Part model, mm, in its own coordinate system. A direction names the side the tool comes from. Round coordinates to 2 decimals unless told otherwise and drop trailing zeros. Loops run counter-clockwise (first coordinate to the right, second up) from the corner with the lowest first, then second, coordinate; pieces in that order, holes last. Notation, with made-up numbers: M 49,84 L 90,84 A13 cw 90,106 Z; hole C 67.25,84 d2. An arc over 180 degrees is marked long. Answer as CSV lines item,"result". Start each with the question number.
Item 1: Band-saw the part on B-B (z = -58). Give the cut face in (x, y), and give its area (3 significant figures).
Item 2: Band-saw the part on A-A (y = 0.95). Count the separate pieces of the cut face and the enclosed holes in it, and give its area (3 significant figures).
Item 3: Which spindle directions (+Z, -Z, +X, -X, +Y, -Y) get a long thin tool onto all of the face, cutting with end or side? Do faces 1 (the flat face through (-8.235, 0, -93)), 2 (the flat face through (0, -1.984, -115)), 3 (the flat face through (8.235, 0, -107)). Say none if no direction does.
Item 4: Wall check: line 1 (Z direction, x = -4.5, y = 0.2); line 2 (Z direction, x = 1, y = 0.6); line 3 (X direction, y = 1.45, z = -103). Give the ranges that are in metal, low to high.
Item 5: Drop flat-ended pins along their axis: pin 1 Ø2 at (y, z) = (0.5, -190.5) entering from -X; pin 2 Ø1.5 at (y, z) = (0.5, -86) entering from -X; pin 3 Ø2 at (x, y) = (2.5, 0.5) entering from -Z. Give the stop position or say it passes through.
```python
from build123d import *

# Parameters (mm, degrees)
BOSS_EXTRUDE1_DEPTH = 1.984375
FILLET1_R           = 17.779999999999998
FILLET3_R           = 2.54


with BuildPart() as part:
    # Sketch1 → Boss-Extrude1 (new, symmetric)
    # profile 1 of 7: a face of its own
    with BuildSketch(Plane(origin=(0, 0, 0), x_dir=(1, 0, 0), z_dir=(0, 1, 0))):
        with BuildLine():
            Line((-8.23515625000002, 7.14375), (0, 7.14375))
            Line((0, 7.14375), (0, 20.43906250000001))
            ThreePointArc((-1.513e-14, 20.43906250000001), (-1.2898437499999995, 21.72890625000001), (-1.567e-14, 23.018750000000008))
            Line((0, 23.018750000000008), (0, 40.48125000000001))
            ThreePointArc((6.485e-14, 40.48125000000001), (-1.984375, 42.46562500000001), (6.445e-14, 44.45000000000001))
            Line((0, 44.45000000000001), (0, 179.38750000000002))
            ThreePointArc((3.455e-13, 179.38750000000002), (-4.295498058784434, 180.01216679408725), (-8.235156249999983, 181.83441966156948))
            Line((-8.235156250000001, 181.83441966156946), (-8.235156250000022, 7.143750000000011))
        make_face()
    # profile 2 of 7: a face of its own
    with BuildSketch(Plane(origin=(0, 0, 0), x_dir=(1, 0, 0), z_dir=(0, 1, 0))):
        with BuildLine():
            Line((0, 20.43906250000001), (0, 7.14375))
            Line((0, 7.14375), (8.23515625000002, 7.14375))
            add(Edge.make_bspline(
                [(8.235156250000017, 40.44394804447435), (6.159687598359963, 38.37781946383395), (8.44847607791561, 34.0776706590483), (3.312171002640199, 23.23056643102504), (2.7641627847252086, 13.194656625268534), (8.23515625000002, 7.143749999999999)],
                knots=[0, 0, 0, 0, 0.20223780839821387, 0.3558357267481405, 1, 1, 1, 1], degree=3))
            Line((8.235156250000017, 40.443948044474354), (8.235156250000001, 181.83441966156946))
            ThreePointArc((8.23515624999998, 181.83441966156948), (4.295498058784762, 180.01216679408734), (3.455e-13, 179.38750000000002))
            Line((0, 179.38750000000002), (0, 44.45000000000001))
            ThreePointArc((6.445e-14, 44.45000000000001), (1.4031650189170781, 43.86879001891704), (1.984375, 42.46562500000001))
            ThreePointArc((1.984375, 42.46562500000001), (1.4031650189170788, 41.06245998108298), (6.485e-14, 40.48125000000001))
            Line((0, 40.48125000000001), (0, 23.018750000000008))
            ThreePointArc((-1.567e-14, 23.018750000000008), (0.9120572622960801, 22.6409635122961), (1.2898437499999995, 21.72890625000001))
            ThreePointArc((1.2898437499999995, 21.72890625000001), (0.9120572622960798, 20.816848987703917), (-1.513e-14, 20.43906250000001))
        make_face()
    # profile 3 of 7: a face of its own
    with BuildSketch(Plane(origin=(0, 0, 0), x_dir=(1, 0, 0), z_dir=(0, 1, 0))):
        Polygon((-8.23515625000002, 7.14375), (0, -8.9e-16), (0, 7.14375), align=None)
    # profile 4 of 7: a face of its own
    with BuildSketch(Plane(origin=(0, 0, 0), x_dir=(1, 0, 0), z_dir=(0, 1, 0))):
        Polygon((0, 7.14375), (0, 0), (8.23515625000002, 7.14375), align=None)
    # profile 5 of 7: a face of its own
    with BuildSketch(Plane(origin=(0, 0, 0), x_dir=(1, 0, 0), z_dir=(0, 1, 0))):
        with BuildLine():
            ThreePointArc((-15.081249999999988, 194.46875), (-13.259723823628677, 187.2837777882518), (-8.235156249999983, 181.83441966156948))
            ThreePointArc((-8.235156249999983, 181.83441966156948), (-4.295498058784434, 180.01216679408725), (3.455e-13, 179.38750000000002))
            Line((0, 179.38750000000002), (0, 190.5))
            ThreePointArc((3.1e-14, 190.5), (-3.96874999999999, 194.46875), (3.197e-14, 198.4375))
            Line((0, 198.4375), (0, 209.54999999999998))
            ThreePointArc((9.2e-16, 209.54999999999998), (-1.1963495653314102, 209.50247373299547), (-2.3851589030460536, 209.3601944755947))
            ThreePointArc((-2.3851589030460536, 209.3601944755947), (-11.476394888401645, 204.2532511077708), (-15.081249999999988, 194.46875))
        make_face()
        with BuildLine():
            Line((-7.717407604043602, 188.99640642622387), (-6.454559087018252, 190.25925494324918))
            ThreePointArc((-6.45455908701825, 190.25925494324918), (-4.209495056750905, 190.25925494324918), (-4.20949505675094, 188.01419091298183))
            Line((-4.209495056750945, 188.01419091298183), (-5.472343573776267, 186.7513423959565))
            ThreePointArc((-5.472343573776268, 186.7513423959565), (-7.717407604043627, 186.75134239595653), (-7.717407604043606, 188.99640642622387))
        make_face(mode=Mode.SUBTRACT)
        with BuildLine():
            Line((-5.472343573776115, 202.1861576040435), (-4.209495056750815, 200.92330908701817))
            ThreePointArc((-4.209495056750815, 200.92330908701817), (-4.209495056750835, 198.67824505675082), (-6.454559087018169, 198.67824505675088))
            Line((-6.454559087018169, 198.67824505675088), (-7.717407604043481, 199.94109357377621))
            ThreePointArc((-7.717407604043492, 199.94109357377621), (-7.717407604043447, 202.18615760404353), (-5.472343573776121, 202.1861576040435))
        make_face(mode=Mode.SUBTRACT)
    # profile 6 of 7: a face of its own
    with BuildSketch(Plane(origin=(0, 0, 0), x_dir=(1, 0, 0), z_dir=(0, 1, 0))):
        with BuildLine():
            Line((0, 190.5), (0, 179.38750000000002))
            ThreePointArc((3.455e-13, 179.38750000000002), (4.295498058784762, 180.01216679408734), (8.23515624999998, 181.83441966156948))
            ThreePointArc((8.23515624999998, 181.83441966156948), (13.259723823628674, 187.2837777882518), (15.081249999999988, 194.46875))
            ThreePointArc((15.081249999999988, 194.46875), (10.664054143769611, 205.13280414376962), (9.2e-16, 209.54999999999998))
            Line((0, 209.54999999999998), (0, 198.4375))
            ThreePointArc((3.197e-14, 198.4375), (2.8063300378341145, 197.2750800378341), (3.96874999999999, 194.46875))
            ThreePointArc((3.96874999999999, 194.46875), (2.806330037834115, 191.6624199621659), (3.1e-14, 190.5))
        make_face()
        with BuildLine():
            ThreePointArc((4.209495056750873, 188.0141909129818), (4.209495056750863, 190.25925494324915), (6.454559087018207, 190.25925494324912))
            Line((6.454559087018202, 190.25925494324912), (7.717407604043522, 188.99640642622379))
            ThreePointArc((7.717407604043532, 188.99640642622379), (7.717407604043521, 186.75134239595644), (5.472343573776178, 186.75134239595644))
            Line((5.472343573776174, 186.75134239595644), (4.209495056750864, 188.0141909129818))
        make_face(mode=Mode.SUBTRACT)
        with BuildLine():
            Line((7.717407604043602, 199.9410935737761), (6.454559087018252, 198.6782450567508))
            ThreePointArc((6.454559087018261, 198.6782450567508), (4.209495056750886, 198.67824505675077), (4.209495056750962, 200.92330908701814))
            Line((4.209495056750945, 200.92330908701817), (5.472343573776294, 202.18615760404347))
            ThreePointArc((5.472343573776303, 202.18615760404347), (7.7174076040436335, 202.18615760404342), (7.717407604043618, 199.94109357377607))
        make_face(mode=Mode.SUBTRACT)
    # profile 7 of 7: a face of its own
    with BuildSketch(Plane(origin=(0, 0, 0), x_dir=(1, 0, 0), z_dir=(0, 1, 0))):
        with BuildLine():
            add(Edge.make_bspline(
                [(-15.081249999999988, 194.46875), (-15.572644055765616, 225.099567963449), (-2.385158903046056, 209.3601944755947)],
                knots=[0, 0, 0, 1, 1, 1], degree=2))
            ThreePointArc((-15.081249999999988, 194.46875), (-11.476394888401645, 204.2532511077708), (-2.3851589030460536, 209.3601944755947))
        make_face()
    extrude(amount=BOSS_EXTRUDE1_DEPTH, both=True)

    # Fillet1
    fillet1_edges = [part.edges().sort_by_distance(p)[0] for p in [
        (-8.235156249999992, 0, -181.83441966156948),
        (8.235156249999992, 0, -181.83441966156948),
    ]]
    fillet(fillet1_edges, radius=FILLET1_R)

    # Fillet3
    fillet3_edges = [part.edges().sort_by_distance(p)[0] for p in [
        (8.235156250000017, -0.9921875, -40.443948044474354),
        (-8.23515625000002, 0, -7.143750000000006),
        (0, 0, 4.4e-16),
        (8.23515625000002, 0.9921875, -7.143749999999999),
    ]]
    fillet(fillet3_edges, radius=FILLET3_R)


solid = part.part
```
Answer block:
1,outline,"M -8.24,-1.98 L 8.24,-1.98 L 8.24,1.98 L -8.24,1.98 Z"
1,area,"65.4 mm^2"
2,separate pieces,"1"
2,enclosed holes,"7"
2,area,"3,510 mm^2"
3,face 1,"+Z, -X, +Y, -Y"
3,face 2,"+Z, -Z, +X, -X, -Y"
3,face 3,"+Z, +X, +Y, -Y"
4,line 1,"z = -211.67 to -201.21, -198.45 to -190.49, -187.72 to -3.9"
4,line 2,"z = -209.52 to -198.31, -190.63 to -44.18, -40.75 to -22.54, -20.91 to -1.03"
4,line 3,"x = -8.24 to 8.24"
5,pin 1,"stops at x = -14.79"
5,pin 2,"stops at x = -8.24"
5,pin 3,"stops at z = -209.48"
